Work out the finished part from the listing and answer in its coordinate system (mm). Round coordinates to 2 decimals unless told otherwise and drop trailing zeros. Order: outer loops, then holes, each group sorted by start corner. A loop starts at its lowest first (then second) coordinate and runs counter-clockwise, first axis right, second up. Notation, with made-up numbers: (34.5, 1.25) -> (57.5, 1.25) arc R21 cw to (57.5, 17.25) -> close; hole circle Ø6 at (20.5, -8.5). An arc over 180 degrees is marked (long way). Use one line per item in the form item = value.
```python
from build123d import *

# Parameters (mm, degrees)
SKETCH1_W           = 64
SKETCH1_H           = 56
SKETCH1_R           = 2
BOSS_EXTRUDE1_DEPTH = 4
SKETCH2_R           = 6.75
CUT_EXTRUDE1_DEPTH  = 4
SKETCH3_R           = 2
CUT_EXTRUDE2_DEPTH  = 4


with BuildPart() as part:
    # Sketch1 → Boss-Extrude1 (new body)
    with BuildSketch(Plane.XY):
        Rectangle(SKETCH1_W, SKETCH1_H)
        with Locations((-12, 23)):
            Circle(SKETCH1_R, mode=Mode.SUBTRACT)
        with Locations((12, 23)):
            Circle(SKETCH1_R, mode=Mode.SUBTRACT)
        with Locations((-12, -23)):
            Circle(SKETCH1_R, mode=Mode.SUBTRACT)
        with Locations((12, -23)):
            Circle(SKETCH1_R, mode=Mode.SUBTRACT)
    extrude(amount=BOSS_EXTRUDE1_DEPTH)

    # Sketch2 → Cut-Extrude1 (cut)
    with BuildSketch(Plane(origin=(0, 0, 0), x_dir=(-1, 0, 0), z_dir=(0, 0, -1))):
        Circle(SKETCH2_R)
    extrude(amount=-CUT_EXTRUDE1_DEPTH, mode=Mode.SUBTRACT)

    # Sketch3 → Cut-Extrude2 (cut)
    with BuildSketch(Plane(origin=(0, 0, 0), x_dir=(-1, 0, 0), z_dir=(0, 0, -1))):
        with Locations((-22, 0)):
            Circle(SKETCH3_R)
        with Locations((22, 0)):
            Circle(SKETCH3_R)
    extrude(amount=-CUT_EXTRUDE2_DEPTH, mode=Mode.SUBTRACT)


solid = part.part
```
Item 1: Determine the mould class of faces 1 (the flat face through (32, 0, 2)), 2 (the flat face through (-32, 0, 2)), 3 (the cylindrical face through (-13.474, -21.648, 1.972)) for opening direction X: released by +X, released by -X, zero draft, split by the parting line, or undercut.
Findings:
face_1 = released by +X
face_2 = released by -X
face_3 = undercut
Item 2: The part is cut by section B-B, the plane y = 0. Give the vertices of the cut face in (x, z).
Findings:
outline = (-32, 0) -> (-24, 0) -> (-24, 4) -> (-32, 4) -> close; (-20, 0) -> (-6.75, 0) -> (-6.75, 4) -> (-20, 4) -> close; (6.75, 0) -> (20, 0) -> (20, 4) -> (6.75, 4) -> close; (24, 0) -> (32, 0) -> (32, 4) -> (24, 4) -> close
Item 3: The part is cut by section A-A, the plane x = 0. Give the vertices of the cut face in (y, z), and give its area (3 significant figures).
Findings:
outline = (-28, 0) -> (-6.75, 0) -> (-6.75, 4) -> (-28, 4) -> close; (6.75, 0) -> (28, 0) -> (28, 4) -> (6.75, 4) -> close
area = 170 mm^2
Item 4: Consider line 1 along Y through (x, z) = (-12, 1.25); line 2 along X through (y, z) = (-22, 0.25); line 3 along X through (y, z) = (0.5, 3.7). Determine where each line is inside the solid, lowest interval first.
Findings:
line_1 = -28 to -25, -21 to 21, 25 to 28
line_2 = -32 to -13.73, -10.27 to 10.27, 13.73 to 32
line_3 = -32 to -23.94, -20.06 to -6.73, 6.73 to 20.06, 23.94 to 32
Item 5: The part is cut by section C-C, the plane z = 1. Give the vertices of the cut face in (x, y), and give its area (3 significant figures).
Findings:
outline = (-32, -28) -> (32, -28) -> (32, 28) -> (-32, 28) -> close; hole circle Ø4 at (-22, 0); hole circle Ø4 at (-12, -23); hole circle Ø4 at (-12, 23); hole circle Ø13.5 at (0, 0); hole circle Ø4 at (12, -23); hole circle Ø4 at (12, 23); hole circle Ø4 at (22, 0)
area = 3,370 mm^2
Item 6: The part is cut by section D-D, the plane y = 23. Give the vertices of the cut face in (x, z), and give its area (3 significant figures).
Findings:
outline = (-32, 0) -> (-14, 0) -> (-14, 4) -> (-32, 4) -> close; (-10, 0) -> (10, 0) -> (10, 4) -> (-10, 4) -> close; (14, 0) -> (32, 0) -> (32, 4) -> (14, 4) -> close
area = 224 mm^2
